from build123d import *

# Parameters (mm, degrees)
EXTRUDE1_DEPTH            = 25.4
F_4_40_TAPPED_HOLE1_D     = 2.2606
F_4_40_TAPPED_HOLE1_DEPTH = 7.5946
F_4_40_TAPPED_HOLE1_TIP   = 0.679152758
F_4_40_TAPPED_HOLE2_D     = 2.2606
F_4_40_TAPPED_HOLE2_DEPTH = 7.5946
F_4_40_TAPPED_HOLE2_TIP   = 0.679152758


with BuildPart() as part:
    # Sketch2 → Extrude1 (new body)
    with BuildSketch(Plane.XY):
        Polygon((-1.833087105, 3.175), (1.833087105, 3.175), (3.666174209, 0), (1.833087105, -3.175), (-1.833087105, -3.175), (-3.666174209, 0), align=None)
    extrude(amount=-EXTRUDE1_DEPTH)

    # #4-40 Tapped Hole1
    with Locations(Plane.XY):
        with Locations((0, 0)):
            Hole(F_4_40_TAPPED_HOLE1_D / 2, depth=F_4_40_TAPPED_HOLE1_DEPTH)
            with Locations((0, 0, -(F_4_40_TAPPED_HOLE1_DEPTH + F_4_40_TAPPED_HOLE1_TIP / 2))):  # 118° drill point
                Cone(0, F_4_40_TAPPED_HOLE1_D / 2, F_4_40_TAPPED_HOLE1_TIP, mode=Mode.SUBTRACT)

    # #4-40 Tapped Hole2
    with Locations(Plane(origin=(0, 0, -25.4), x_dir=(-1, 0, 0), z_dir=(0, 0, -1))):
        with Locations((0, 0)):
            Hole(F_4_40_TAPPED_HOLE2_D / 2, depth=F_4_40_TAPPED_HOLE2_DEPTH)
            with Locations((0, 0, -(F_4_40_TAPPED_HOLE2_DEPTH + F_4_40_TAPPED_HOLE2_TIP / 2))):  # 118° drill point
                Cone(0, F_4_40_TAPPED_HOLE2_D / 2, F_4_40_TAPPED_HOLE2_TIP, mode=Mode.SUBTRACT)


solid = part.part
The model under review builds one solid part; all positions refer to its coordinate system, in mm. A direction names the side the tool comes from. Give positions to 0.01 mm unless a question says otherwise; leave off trailing zeros. Write each loop counter-clockwise with the first axis right and the second up, starting at its lowest first coordinate (ties: lowest second). Pieces come first, ordered by that corner, then holes.
1. Tool access review of faces 4 (the flat face through (2.76, -1.57, -12.52)), 5 (the cylindrical face through (0.245, -1.103, -3.85)), 6 (the cylindrical face through (-0.245, -1.103, -21.55)): name each direction out of +Z, -Z, +X, -X, +Y, -Y from which nothing blocks a thin tool from reaching the whole face with its end or side.
2. Wall thickness on L1, parallel to Y at x = 0, z = -5.5 (3 decimals); L2, parallel to X at y = 0.75, z = -7.5; L3, parallel to X at y = -0.25, z = -5.75: over which ranges is each line inside the solid? List them lowest first.
3. Draft analysis for pull direction Y (two halves, no side actions). For faces 1 (the flat face through (0, -3.175, -13)), 2 (the conical face through (0.043, -0.192, -17.244)), 3 (the flat face through (-2.76, 1.57, -12.52)), state which applies: +Y half, -Y half, draft (parallel to the pull), parting line (faces both ways), or undercut.
4. Add section B-B, the plane y = -1.75. Write out the cut boundary in (x, z).
5. For P1, Ø2, axis at x = 0, y = 0, coming from the -Z side; P2, Ø1.4, axis at x = 0, y = 0, coming from the +Z side, all flat-tipped, find the tip position at first contact; note any pin that passes through.
6. Add section C-C, the plane z = -8. Write out the cut boundary in (x, y) (3 decimals), plus the area to 3 significant figures.
7. Add section A-A, the plane z = -20.5. Write out the cut boundary in (x, y) (3 decimals).
8. Add section D-D, the plane y = 2.5. Write out the cut boundary in (x, z).
Worked answers:
1. face 4: +Z, -Z, +X, -Y
1. face 5: +Z
1. face 6: -Z
2. L1: y = -3.175 to -1.13, 1.13 to 3.175
2. L2: x = -3.23 to -0.85, 0.85 to 3.23
2. L3: x = -3.52 to -1.1, 1.1 to 3.52
3. face 1: -Y half
3. face 2: undercut
3. face 3: +Y half
4. outline: (-2.66, -25.4) - (2.66, -25.4) - (2.66, 0) - (-2.66, 0) - close
5. P1: stops at z = -17.73
5. P2: stops at z = -7.85
6. outline: (-3.666, 0) - (-1.833, -3.175) - (1.833, -3.175) - (3.666, 0) - (1.833, 3.175) - (-1.833, 3.175) - close; hole circle Ø0.911 at (0, 0)
6. area: 34.3 mm2
7. outline: (-3.666, 0) - (-1.833, -3.175) - (1.833, -3.175) - (3.666, 0) - (1.833, 3.175) - (-1.833, 3.175) - close; hole circle Ø2.261 at (0, 0)
8. outline: (-2.22, -25.4) - (2.22, -25.4) - (2.22, 0) - (-2.22, 0) - close
